```python
from build123d import *

# Parameters (mm, degrees)
F1_DEPTH = 20
F2_W     = 4
F2_H     = 12
F3_DEPTH = 59
F4_W     = 6
F4_H     = 2
F5_DEPTH = 39
F6_R     = 1.3
F7_DEPTH = 7.3


with BuildPart() as f1:
    # F0 (on Top) → F1 (new body)
    with BuildSketch(Plane.XY):
        with BuildLine():
            ThreePointArc((0, 4.05), (4.05, 0), (0, -4.05))
            Line((0, -4.05), (-6.35, -4.05))
            Line((-6.35, -4.05), (-6.35, -14))
            Line((-6.35, -14), (6.35, -14))
            Line((6.35, -14), (6.35, 12))
            Line((6.35, 12), (18.05, 12))
            Line((18.05, 12), (18.05, 55.5))
            Line((18.05, 55.5), (6.35, 55.5))
            Line((6.35, 55.5), (4.05, 55.5))
            Line((4.05, 55.5), (4.05, 44))
            ThreePointArc((4.05, 44), (0, 39.95), (-4.05, 44))
            Line((-4.05, 44), (-4.05, 55.5))
            Line((-4.05, 55.5), (-6.35, 55.5))
            Line((-6.35, 55.5), (-6.35, 33.5))
            Line((-6.35, 33.5), (2.15, 33.5))
            Line((2.15, 33.5), (2.15, 32.5))
            Line((2.15, 32.5), (2.15, 9.35))
            Line((2.15, 9.35), (-6.35, 9.35))
            Line((-6.35, 9.35), (-6.35, 4.05))
            Line((-6.35, 4.05), (0, 4.05))
        make_face()
    extrude(amount=F1_DEPTH)

    # F2 (on face) → F3 (cut)
    with BuildSketch(Plane(origin=(0, 55.5, 0), x_dir=(-1, 0, 0), z_dir=(0, 1, 0))):
        with Locations((-11.05, 10)):
            Rectangle(F2_W, F2_H)
    extrude(amount=-F3_DEPTH, mode=Mode.SUBTRACT)

    # F4 (on face) → F5 (cut)
    with BuildSketch(Plane.XZ.offset(-12)):
        Polygon((15.05, 16), (9.05, 16), (9.05, 10), (9.05, 4), (15.05, 4), align=None)
        with Locations((12.05, 3)):
            Rectangle(F4_W, F4_H)
        with Locations((12.05, 17)):
            Rectangle(F4_W, F4_H)
    extrude(amount=-F5_DEPTH, mode=Mode.SUBTRACT)

    # F6 (on face) → F7 (cut)
    with BuildSketch(Plane.YZ.offset(18.05)):
        with Locations((47.75, 10)):
            Circle(F6_R)
        with Locations((19.75, 10)):
            Circle(F6_R)
    extrude(amount=-F7_DEPTH, mode=Mode.SUBTRACT)


solid = f1.part
```
The model under review builds one solid part; all positions refer to its coordinate system, in mm. A direction names the side the tool comes from. Round coordinates to 2 decimals unless told otherwise and drop trailing zeros. Write each loop counter-clockwise with the first axis right and the second up, starting at its lowest first coordinate (ties: lowest second). Pieces come first, ordered by that corner, then holes.
(1) We need section C-C on z = 10. Give the number of separate pieces and of enclosed holes in the cut face, and give its area (3 significant figures).
(2) Machinability: for faces 1 (the flat face through (11, 53, 4)), 2 (the flat face through (6.35, -1, 10)), 3 (the flat face through (9.05, 34, 10)), 4 (the flat face through (2.15, 22, 10)), 5 (the flat face through (6, 29, 20)), which of the approach directions +Z, -Z, +X, -X, +Y, -Y give a long, thin tool a straight path to every point of the face, cutting with its end or side? Answer none if there is none.
(3) We need section D-D on x = 16. Give the boundary of the cut face in (y, z), and give its area (3 significant figures).
(4) Insertion check: pin 1 (12 mm diameter, centred on x = 11, z = 17.5, fed in from -Y); pin 2 (2 mm diameter, centred on x = 10, z = 16, fed in from -Y); pin 3 (3 mm diameter, centred on y = 19.75, z = 10, fed in from -X); pin 4 (7 mm diameter, centred on x = 0, z = 5, fed in from +Y). Each pin has a flat end and moves straight along its axis. Give the tip position at first contact, or say it passes through.
(5) Mouldability with a two-part tool opening along Y and no side actions: class faces 6 (the flat face through (-3, -4.05, 10)), 7 (the flat face through (8, 12, 10)), 8 (the flat face through (12, 31, 2)) as +Y half, -Y half, draft (parallel to the pull), parting line (faces both ways), or undercut.
(6) We need section B-B on z = 4.75. Give the boundary of the cut face in (x, y), and give its area (3 significant figures).
(7) We need section A-A on y = 47.75. Give the boundary of the cut face in (x, z).
(8) Wall thickness on L1, parallel to X at y = 49, z = 6.75; L2, parallel to X at y = 30, z = 15.25; L3, parallel to X at y = 35.5, z = 16.5: over which ranges is each line inside the solid? List them lowest first.
Findings below:
1. separate pieces: 4
1. enclosed holes: 0
1. area: 723 mm2
2. face 1: +Y, -Y
2. face 2: +Z, -Z, +X, -Y
2. face 3: -Y
2. face 4: +Z, -Z, -X
2. face 5: +Z, +X, -X, +Y, -Y
3. outline: (12, 0) - (55.5, 0) - (55.5, 20) - (12, 20) - close; hole circle Ø2.6 at (19.75, 10); hole circle Ø2.6 at (47.75, 10)
3. area: 859 mm2
4. pin 1: stops at y = -14
4. pin 2: stops at y = 12
4. pin 3: stops at x = 2.15
4. pin 4: stops at y = 41.96
5. face 6: undercut
5. face 7: -Y half
5. face 8: draft
6. outline: (-6.35, -14) - (6.35, -14) - (6.35, 12) - (9.05, 12) - (9.05, 55.5) - (4.05, 55.5) - (4.05, 44) arc R4.05 cw to (-4.05, 44) - (-4.05, 55.5) - (-6.35, 55.5) - (-6.35, 33.5) - (2.15, 33.5) - (2.15, 9.35) - (-6.35, 9.35) - (-6.35, 4.05) - (0, 4.05) arc R4.05 cw to (0, -4.05) - (-6.35, -4.05) - close; (13.05, 51) - (15.05, 51) - (15.05, 12) - (18.05, 12) - (18.05, 55.5) - (13.05, 55.5) - close
6. area: 738 mm2
7. outline: (-6.35, 0) - (-4.05, 0) - (-4.05, 20) - (-6.35, 20) - close; (4.05, 0) - (18.05, 0) - (18.05, 8.7) - (15.05, 8.7) - (15.05, 2) - (9.05, 2) - (9.05, 18) - (15.05, 18) - (15.05, 11.3) - (18.05, 11.3) - (18.05, 20) - (4.05, 20) - close
8. L1: x = -6.35 to -4.05, 4.05 to 9.05, 15.05 to 18.05
8. L2: x = 2.15 to 9.05, 15.05 to 18.05
8. L3: x = -6.35 to 9.05, 15.05 to 18.05
